The model under review builds one solid part; all positions refer to its coordinate system, in mm. Face numbers are marked on the shaded views. A direction names the side the tool comes from. Coordinates: 2 decimals unless noted, no trailing zeros. Order: outer loops, then holes, each group sorted by start corner. A loop starts at its lowest first (then second) coordinate and runs counter-clockwise, first axis right, second up.
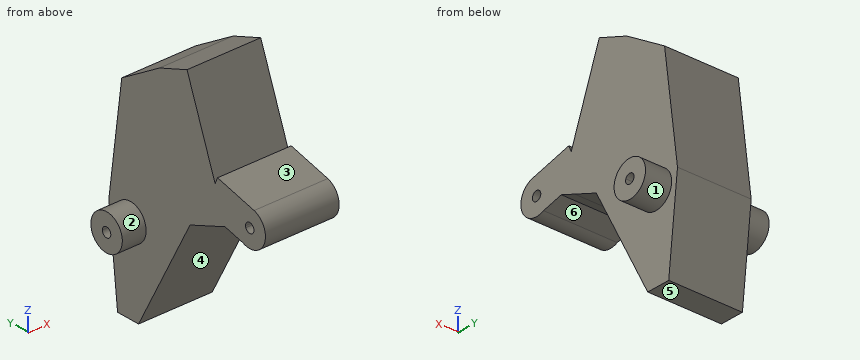
```python
from build123d import *

# Parameters (mm, degrees)
F3_DEPTH      = 15
F3_DEPTH_BACK = 16
F4_DEPTH      = 26
F4_DEPTH_BACK = 26
F6_DEPTH      = 25
F6_DEPTH_BACK = 25


# Not quite as in the source:
# - a feature names something its author has since deleted; it is built from what else it names


with BuildPart() as f3:
    # F0 (on Right) → F3 (new body, two sides)
    with BuildSketch(Plane.YZ) as f3_sk:
        Polygon((42.99440903, 39.7499332097), (24.4999610724, -9.4537481835), (28.4550828122, -10.9799026477), (53, -57.2503693402), (63, -57.2503693402), (67.1839944136, -18.0194567546), (61.0229901087, 28.5260152414), align=None)
        with BuildLine():
            ThreePointArc((64.4101656244, -21.9598052953), (55.5369643161, -29.3330215655), (49.9130141132, -19.2598292344))
            ThreePointArc((49.9130141132, -19.2598292344), (58.2833669326, -14.5865890251), (64.4101656244, -21.9598052953))
        make_face(mode=Mode.SUBTRACT)
        with BuildLine():
            Line((3.3187451802, -6.7257661592), (11.7920777761, -4.5501841217))
            Line((11.7920777761, -4.5501841217), (18.186862473, -7.0177261735))
            Line((18.186862473, -7.0177261735), (24.4999610724, -9.4537481835))
            Line((24.4999610724, -9.4537481835), (42.99440903, 39.7499332097))
            Line((42.99440903, 39.7499332097), (28.0174564582, 45.3793995842))
            Line((28.0174564582, 45.3793995842), (15.3511571156, 11.6812562976))
            Line((15.3511571156, 11.6812562976), (-2.0833397847, 7.2048383286))
            ThreePointArc((-2.0833397847, 7.2048383286), (-6.9926384128, -2.7116430495), (3.3187451802, -6.7257661592))
        make_face()
        with BuildLine():
            ThreePointArc((2, 0), (1.9661910054, -0.3661870155), (1.8659070697, -0.7199936162))
            ThreePointArc((1.8659070697, -0.7199936162), (-1.9661910054, 0.3661870155), (2, 0))
        make_face(mode=Mode.SUBTRACT)
    extrude(amount=F3_DEPTH)
    extrude(f3_sk.sketch, amount=-F3_DEPTH_BACK)

    # F0 (on Right) → F4 (join, two sides)
    with BuildSketch(Plane.YZ) as f4_sk:
        with BuildLine():
            ThreePointArc((64.4101656244, -21.9598052953), (58.2833669326, -14.5865890251), (49.9130141132, -19.2598292344))
            ThreePointArc((49.9130141132, -19.2598292344), (55.5369643161, -29.3330215655), (64.4101656244, -21.9598052953))
        make_face()
        with BuildLine():
            ThreePointArc((58.9101656244, -21.9598052953), (56.5439786088, -23.9259963007), (55.0442585547, -21.2398116791))
            ThreePointArc((55.0442585547, -21.2398116791), (57.2763526399, -19.9936142899), (58.9101656244, -21.9598052953))
        make_face(mode=Mode.SUBTRACT)
    extrude(amount=F4_DEPTH)
    extrude(f4_sk.sketch, amount=-F4_DEPTH_BACK)

    # F5 (on Right) → F6 (cut, two sides)
    with BuildSketch(Plane.YZ) as f6_sk:
        Polygon((16.4947576102, 9.0393807374), (29.8895755297, 44.6757162874), (28.0174564582, 45.3793995842), (15.3511571156, 11.6812562976), align=None)
    extrude(amount=-F6_DEPTH, mode=Mode.SUBTRACT)
    extrude(f6_sk.sketch, amount=F6_DEPTH_BACK, mode=Mode.SUBTRACT)


solid = f3.part
```
(1) Machinability: for the marked faces 1, 2 and 3, which of the approach directions +Z, -Z, +X, -X, +Y, -Y give a long, thin tool a straight path to every point of the face, cutting with its end or side? Answer none if there is none.
A:
face 1: +X
face 2: -X
face 3: +Z, +X, -X, -Y
(2) We need section A-A, the plane x = 6.5. Write out the cut boundary in (y, z), and give its area (3 significant figures).
A:
outline: (-2.08, 7.2) arc R7.5 ccw (long way) to (3.32, -6.73) - (11.79, -4.55) - (28.46, -10.98) - (53, -57.25) - (63, -57.25) - (67.18, -18.02) - (61.02, 28.53) - (42.99, 39.75) - (29.89, 44.68) - (16.49, 9.04) - (15.35, 11.68) - close; hole circle Ø4 at (0, 0); hole circle Ø4 at (56.91, -21.96)
area: 3,550 mm2
(3) For pin 1 Ø22.5 at (y, z) = (32, -9) entering from +X; pin 2 Ø1 at (x, y) = (-7.5, 32) entering from -Z; pin 3 Ø4 at (x, z) = (15, 30) entering from -Y, all flat-tipped, find the tip position at first contact; note any pin that passes through.
A:
pin 1: stops at x = 15
pin 2: stops at z = -18.61
pin 3: stops at y = 23.62
(4) We need section C-C, the plane z = 10.5. Write out the cut boundary in (x, y).
A:
outline: (-16, 10.75) - (15, 10.75) - (15, 15.86) - (-16, 15.86) - close; (-16, 17.04) - (15, 17.04) - (15, 63.41) - (-16, 63.41) - close
(5) We need section B-B, the plane y = 0. Write out the cut boundary in (x, z).
A:
outline: (-16, -7.5) - (15, -7.5) - (15, -2) - (-16, -2) - close; (-16, 2) - (15, 2) - (15, 7.74) - (-16, 7.74) - close
(6) Draft analysis for pull direction Y (two halves, no side actions). For the marked faces 4, 5 and 6, state which applies: released by +Y, released by -Y, zero draft, split by the parting line, or undercut.
A:
face 4: released by -Y
face 5: zero draft
face 6: undercut
(7) We need section D-D, the plane x = 22. Write out the cut boundary in (y, z).
A:
outline: circle Ø15 at (56.91, -21.96); hole circle Ø4 at (56.91, -21.96)
(8) Wall thickness on probe 1 along X at (y, z) = (53, -38); probe 2 along Z at (x, y) = (5, 0); probe 3 along Z at (x, y) = (-10.5, 1): over which ranges is each line inside the solid? List them lowest first.
A:
probe 1: x = -16 to 15
probe 2: z = -7.5 to -2, 2 to 7.74
probe 3: z = -7.43 to -1.73, 1.73 to 8
